Model file for the job. Use its own axes, mm. Face numbers are marked on the shaded views. Give positions to 0.01 mm unless a question says otherwise; leave off trailing zeros. Write each loop counter-clockwise with the first axis right and the second up, starting at its lowest first coordinate (ties: lowest second). Pieces come first, ordered by that corner, then holes. Notation, with made-up numbers: (-19.75, 64.25) - (28.25, 64.25) arc R19 ccw to (28.25, 75.25) - close; hole circle Ø9 at (-28, 66.5). An arc over 180 degrees is marked (long way). Use a Markdown table: item, result. Add a question column.
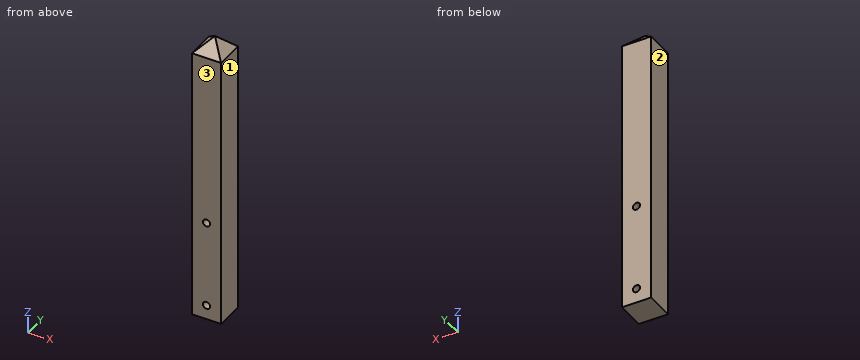
```python
from build123d import *

# Parameters (mm, degrees)
SKETCH1_W           = 20
SKETCH1_H           = 200
SKETCH1_R           = 2.5
BOSS_EXTRUDE1_DEPTH = 20
CHAMFER1_SIZE       = 10


with BuildPart() as part:
    # Sketch1 → Boss-Extrude1 (new body)
    with BuildSketch(Plane(origin=(0, 0, 0), x_dir=(1, 0, 0), z_dir=(0, 1, 0))):
        with Locations((10, -100)):
            Rectangle(SKETCH1_W, SKETCH1_H)
        with Locations(Location((10, -10, 0), (0, 0, 270))):
            Circle(SKETCH1_R, mode=Mode.SUBTRACT)
        with Locations(Location((10, -70, 0), (0, 0, 270))):
            Circle(SKETCH1_R, mode=Mode.SUBTRACT)
    extrude(amount=BOSS_EXTRUDE1_DEPTH)

    # Chamfer1
    chamfer1_edges = [part.edges().sort_by_distance(p)[0] for p in [
        (10, 0, 200),
        (10, 20, 200),
        (20, 10, 200),
        (0, 10, 200),
    ]]
    chamfer(chamfer1_edges, length=CHAMFER1_SIZE - 0.0001)  # a hair under: the kernel refuses the full size


solid = part.part
```
(1) Probe probe 1 along X at (y, z) = (15, 70); probe 2 along Z at (x, y) = (12.25, 15.5); probe 3 along Z at (x, y) = (8, 4.5). List the from-to ranges inside material, lowest first. Write a range as [from, to].
(2) Band-saw the part on D-D (y = 17.75). Write the cut outline in (x, z).
(3) Band-saw the part on A-A (z = 10). Write the cut outline in (x, y), then the cut area to 3 significant figures.
(4) Two-plate mould, pull along X, no slides. Class the marked faces 1, 2 and 3: +X half, -X half, draft (parallel to the pull), parting line (faces both ways), or undercut.
(5) Band-saw the part on B-B (y = 3). Write the cut outline in (x, z).
(6) Band-saw the part on C-C (x = 16). Write the cut outline in (y, z).
(7) Flat gauge pins, fed straight in: pin 1 (6 mm diameter, centred on x = 3.5, y = 7.5, fed in from +Z); pin 2 (6 mm diameter, centred on x = 5, y = 13, fed in from +Z). Where does each tip first touch, or does it go through?
Model answer:
| question | item | result |
|---|---|---|
| 1 | probe 1 | x = [0, 7.5], [12.5, 20] |
| 1 | probe 2 | z = [0, 8.91], [11.09, 68.91], [71.09, 194.5] |
| 1 | probe 3 | z = [0, 8.5], [11.5, 68.5], [71.5, 194.5] |
| 2 | outline | (0, 0) - (20, 0) - (20, 190) - (17.75, 192.25) - (2.25, 192.25) - (0, 190) - close; hole circle Ø5 at (10, 10); hole circle Ø5 at (10, 70) |
| 3 | outline | (0, 0) - (7.5, 0) - (7.5, 20) - (0, 20) - close; (12.5, 0) - (20, 0) - (20, 20) - (12.5, 20) - close |
| 3 | area | 300 mm^2 |
| 4 | face 1 | +X half |
| 4 | face 2 | -X half |
| 4 | face 3 | draft |
| 5 | outline | (0, 0) - (20, 0) - (20, 190) - (17, 193) - (3, 193) - (0, 190) - close; hole circle Ø5 at (10, 10); hole circle Ø5 at (10, 70) |
| 6 | outline | (0, 0) - (20, 0) - (20, 190) - (16, 194) - (4, 194) - (0, 190) - close |
| 7 | pin 1 | stops at z = 196.5 |
| 7 | pin 2 | stops at z = 197.87 |
